Design review of the part built by this model. Coordinates are the model's own, in mm. Face numbers are marked on the shaded views. A direction names the side the tool comes from. Give positions to 0.01 mm unless a question says otherwise; leave off trailing zeros. Loops run counter-clockwise (first coordinate to the right, second up) from the corner with the lowest first, then second, coordinate; pieces in that order, holes last. Notation, with made-up numbers: (43.5, 66) -> (75.5, 66) arc R11 cw to (75.5, 79) -> close; hole circle Ø2 at (4, 65). An arc over 180 degrees is marked (long way). Use CSV: the item, a comma, the result in double quotes. Start each with the question number.
Item 1: We need section B-B (z = 4). State the section outline as (x, y) points, plus the area to 3 significant figures.
Item 2: For the marked faces 4 and 5, list the 3-axis set-ups (+Z, -Z, +X, -X, +Y, -Y) from which the entire face can be reached by the end or side of a thin tool; tool diameter is ignored.
Item 3: The part is to be moulded in two halves that separate along Y. For the marked faces 1, 2 and 3, say which applies: +Y half, -Y half, draft (parallel to the pull), parting line (faces both ways), or undercut.
Item 4: Clearance check with flat-ended pins moving along their axes: pin 1 (1.7 mm diameter, centred on x = -2, z = -13.5, fed in from -Y); pin 2 (4 mm diameter, centred on x = 11.5, z = 23, fed in from +Y); pin 3 (15 mm diameter, centred on x = 24.5, z = 1.5, fed in from -Y); pin 4 (1.7 mm diameter, centred on x = 1.5, z = -12.5, fed in from +Y). State where each tip first meets the part, or that it passes through.
Item 5: We need section C-C (x = 23). State the section outline as (y, z) points.
Item 6: Wall thickness on line 1 along Z through (x, y) = (34, -8.5); line 2 along X through (y, z) = (22.5, -26): over which ranges is each line inside the solid? List them lowest first. Write a range as from..to.
Item 7: We need section A-A (y = -23). State the section outline as (x, z) points, plus the area to 3 significant figures.
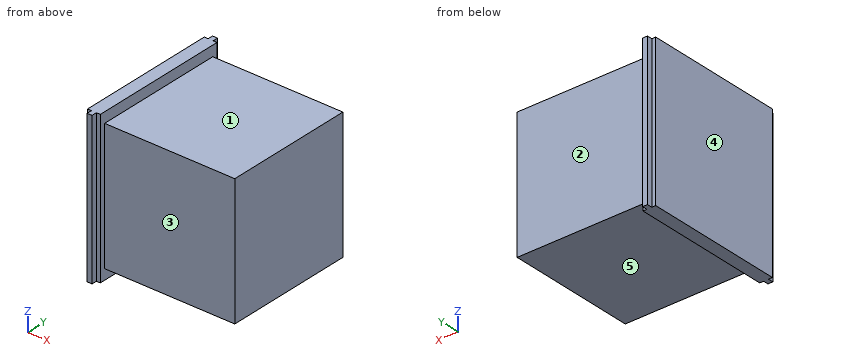
from build123d import *

# Parameters (mm, degrees)
BOX_W     = 50
BOX_H     = 50
BOX_DEPTH = 50
PAD_DEPTH = 29


with BuildPart() as cube:
    # Box → Box (new body)
    with BuildSketch(Plane(origin=(2.45, -25, -25), x_dir=(1, 0, 0), z_dir=(0, 0, 1))):
        with Locations((25, 25)):
            Rectangle(BOX_W, BOX_H)
    extrude(amount=BOX_DEPTH)


with BuildPart() as fusion:
    # Sketch → Pad (new body, symmetric)
    with BuildSketch(Plane.XY):
        Polygon((-2.45, 27), (-0.95, 27), (-0.95, 29), (0.95, 29), (0.95, 27), (2.45, 27), (2.45, 0), (-2.45, 0), align=None)
    pad = extrude(amount=PAD_DEPTH, both=True)

    # Mirrored: Pad across XZ
    add(pad.mirror(Plane.XZ))

    # Fusion: union Cube
    add(cube.part)


solid = fusion.part
Results found:
1,outline,"(-2.45, -27) -> (-0.95, -27) -> (-0.95, -29) -> (0.95, -29) -> (0.95, -27) -> (2.45, -27) -> (2.45, -25) -> (52.45, -25) -> (52.45, 25) -> (2.45, 25) -> (2.45, 27) -> (0.95, 27) -> (0.95, 29) -> (-0.95, 29) -> (-0.95, 27) -> (-2.45, 27) -> close"
1,area,"2,770 mm²"
2,face 4,"+Z, -Z, -X, +Y, -Y"
2,face 5,"-Z, +X, +Y, -Y"
3,face 1,"draft"
3,face 2,"+Y half"
3,face 3,"-Y half"
4,pin 1,"y = -27"
4,pin 2,"y = 25"
4,pin 3,"y = -25"
4,pin 4,"y = 29"
5,outline,"(-25, -25) -> (25, -25) -> (25, 25) -> (-25, 25) -> close"
6,line 1,"-25..25"
6,line 2,"-2.45..2.45"
7,outline,"(-2.45, -29) -> (2.45, -29) -> (2.45, -25) -> (52.45, -25) -> (52.45, 25) -> (2.45, 25) -> (2.45, 29) -> (-2.45, 29) -> close"
7,area,"2,780 mm²"
